The model under review builds one solid part; all positions refer to its coordinate system, in mm. A direction names the side the tool comes from. Round coordinates to 2 decimals unless told otherwise and drop trailing zeros. Loops run counter-clockwise (first coordinate to the right, second up) from the corner with the lowest first, then second, coordinate; pieces in that order, holes last. Notation, with made-up numbers: (25.5, -39) -> (56.5, -39) arc R17 ccw to (56.5, -24) -> close; hole circle Ø9 at (-19.5, 60). An arc over 180 degrees is marked (long way). Return JSON: item names as keys, results as strings. Group by question number.
```python
from build123d import *

# Parameters (mm, degrees)
F1_DEPTH      = 60
F1_DEPTH_BACK = 60
F2_R          = 35
F3_DEPTH      = 43
F3_DEPTH_BACK = 43
F4_R          = 1.9
F5_DEPTH      = 50
F5_DEPTH_BACK = 50


with BuildPart() as f1:
    # F0 (on Front) → F1 (new body, two sides)
    with BuildSketch(Plane.XZ) as f1_sk:
        with BuildLine():
            Line((-39, -19.5), (39, -19.5))
            Line((39, -19.5), (39, 19.5))
            Line((39, 19.5), (26, 19.5))
            ThreePointArc((26, 19.5), (0, -6.5), (-26, 19.5))
            Line((-26, 19.5), (-39, 19.5))
            Line((-39, 19.5), (-39, -19.5))
        make_face()
    extrude(amount=F1_DEPTH)
    extrude(f1_sk.sketch, amount=-F1_DEPTH_BACK)

    # F2 (on Front) → F3 (cut, two sides)
    with BuildSketch(Plane.XZ) as f3_sk:
        with Locations((0, 19.5)):
            Circle(F2_R)
    extrude(amount=-F3_DEPTH, mode=Mode.SUBTRACT)
    extrude(f3_sk.sketch, amount=F3_DEPTH_BACK, mode=Mode.SUBTRACT)

    # F4 (on Top) → F5 (cut, two sides)
    with BuildSketch(Plane.XY) as f5_sk:
        with Locations((-32.2727300227, 51.4772757888)):
            Circle(F4_R)
        with Locations((32.2727300227, 51.4772757888)):
            Circle(F4_R)
        with Locations((32.2727300227, -51.4772757888)):
            Circle(F4_R)
        with Locations((-32.2727300227, -51.4772757888)):
            Circle(F4_R)
    extrude(amount=-F5_DEPTH, mode=Mode.SUBTRACT)
    extrude(f5_sk.sketch, amount=F5_DEPTH_BACK, mode=Mode.SUBTRACT)


solid = f1.part
```
1. We need section A-A, the plane z = -4. Write out the cut boundary in (x, y).
2. Draft analysis for pull direction Y (two halves, no side actions). For faces 1 (the face through (-30.518, -52.205, 0.273)), 2 (the face through (34.03, -52.2, 0.27)), 3 (the face through (35.5, -0.8, 19.5)), 4 (the face through (-1, 60, -8)), state which applies: pulls with the +Y half, pulls with the -Y half, needs draft (parallel to the pull), parting line crosses it, or undercut.
3. Wall thickness on line 1 (Y direction, x = -32, z = -4); line 2 (Y direction, x = -2, z = -10.5); line 3 (Z direction, x = 1, y = -5): over which ranges is each line inside the solid? List them lowest first.
4. We need section B-B, the plane x = 0. Write out the cut boundary in (y, z), then the cut area to 3 significant figures.
5. Tool access review of faces 5 (the face through (-3, 43, -7)), 6 (the face through (-1, -60, -8)): name each direction out of +Z, -Z, +X, -X, +Y, -Y from which nothing blocks a thin tool from reaching the whole face with its end or side.
6. We need section C-C, the plane y = 14.5. Write out the cut boundary in (x, z), then the cut area to 3 significant figures.
7. We need section D-D, the plane z = 11. Write out the cut boundary in (x, y).
Check sheet entries:
{
 "1": {"outline": "(-39, -60) -> (-11.12, -60) -> (-11.12, -43) -> (-25.94, -43) -> (-25.94, 43) -> (-11.12, 43) -> (-11.12, 60) -> (-39, 60) -> close; (11.12, -60) -> (39, -60) -> (39, 60) -> (11.12, 60) -> (11.12, 43) -> (25.94, 43) -> (25.94, -43) -> (11.12, -43) -> close; hole circle Ø3.8 at (-32.27, -51.48); hole circle Ø3.8 at (-32.27, 51.48); hole circle Ø3.8 at (32.27, -51.48); hole circle Ø3.8 at (32.27, 51.48)"},
 "2": {"face 1": "undercut", "face 2": "undercut", "face 3": "needs draft", "face 4": "pulls with the +Y half"},
 "3": {"line 1": "y = -60 to -53.36, -49.6 to 49.6, 53.36 to 60", "line 2": "y = -60 to -43, 43 to 60", "line 3": "z = -19.5 to -15.49"},
 "4": {"outline": "(-60, -19.5) -> (60, -19.5) -> (60, -6.5) -> (43, -6.5) -> (43, -15.5) -> (-43, -15.5) -> (-43, -6.5) -> (-60, -6.5) -> close", "area": "786 mm²"},
 "5": {"face 5": "+Z", "face 6": "+Z, -Z, +X, -X, -Y"},
 "6": {"outline": "(-39, -19.5) -> (39, -19.5) -> (39, 19.5) -> (35, 19.5) arc R35 cw to (-35, 19.5) -> (-39, 19.5) -> close", "area": "1,120 mm²"},
 "7": {"outline": "(-39, -60) -> (-24.57, -60) -> (-24.57, -43) -> (-33.95, -43) -> (-33.95, 43) -> (-24.57, 43) -> (-24.57, 60) -> (-39, 60) -> close; (24.57, -60) -> (39, -60) -> (39, 60) -> (24.57, 60) -> (24.57, 43) -> (33.95, 43) -> (33.95, -43) -> (24.57, -43) -> close; hole circle Ø3.8 at (-32.27, -51.48); hole circle Ø3.8 at (-32.27, 51.48); hole circle Ø3.8 at (32.27, -51.48); hole circle Ø3.8 at (32.27, 51.48)"}
}
